Can you work these out from the model? Positions are in its coordinate system, mm. A direction names the side the tool comes from. Give positions to 0.01 mm unless a question says otherwise; leave off trailing zeros. Write each loop counter-clockwise with the first axis right and the second up, starting at its lowest first coordinate (ties: lowest second). Pieces come first, ordered by that corner, then holes. Notation, with made-up numbers: (62.25, -34) -> (119.25, -34) arc R19 ccw to (119.25, 2) -> close; hole circle Ø7 at (25.25, 2). An arc over 180 degrees is marked (long way). One line per item, written item: value.
from build123d import *

# Parameters (mm, degrees)
SKETCH1_W                                   = 100
SKETCH1_H                                   = 100
BOSS_EXTRUDE1_DEPTH                         = 6.5
SKETCH2_W                                   = 100
SKETCH2_H                                   = 100
BOSS_EXTRUDE2_DEPTH                         = 5
SKETCH3_W                                   = 100
SKETCH3_H                                   = 100
BOSS_EXTRUDE3_DEPTH                         = 5
CUT_EXTRUDE1_DEPTH                          = 101
SKETCH6_W                                   = 100
SKETCH6_H                                   = 100
SKETCH6_W_2                                 = 90
SKETCH6_H_2                                 = 90
CUT_EXTRUDE2_DEPTH                          = 5
SKETCH9_W                                   = 70
SKETCH9_H                                   = 70
BOSS_EXTRUDE4_DEPTH                         = 3.5
CBORE_FOR_M5_CHEESE_HEAD_SCREW1_D           = 3.332
CBORE_FOR_M5_CHEESE_HEAD_SCREW1_DEPTH       = 11
CBORE_FOR_M5_CHEESE_HEAD_SCREW1_CBORE_D     = 8
CBORE_FOR_M5_CHEESE_HEAD_SCREW1_CBORE_DEPTH = 5
CBORE_FOR_M5_CHEESE_HEAD_SCREW1_TIP         = 1.001033791
FILLET1_R                                   = 6.35
CHAMFER1_SIZE                               = 6.35
SKETCH14_W                                  = 25
SKETCH14_H                                  = 50
CUT_EXTRUDE3_DEPTH                          = 5


with BuildPart() as part:
    # Sketch1 → Boss-Extrude1 (new body)
    with BuildSketch(Plane(origin=(0, 0, 0), x_dir=(1, 0, 0), z_dir=(0, 1, 0))):
        Rectangle(SKETCH1_W, SKETCH1_H)
    extrude(amount=BOSS_EXTRUDE1_DEPTH)



with BuildPart() as body_2:
    # Sketch2 → Boss-Extrude2 (new body)
    with BuildSketch(Plane(origin=(0, -3.5, 0), x_dir=(-1, 0, 0), z_dir=(0, -1, 0))):
        Rectangle(SKETCH2_W, SKETCH2_H)
    extrude(amount=BOSS_EXTRUDE2_DEPTH)

    # Sketch3 → Boss-Extrude3 (add)
    with BuildSketch(Plane.XZ.offset(8.5)):
        Rectangle(SKETCH3_W, SKETCH3_H)
    extrude(amount=BOSS_EXTRUDE3_DEPTH)

    # Sketch4 → Cut-Extrude1 (cut, through all)
    with BuildSketch(Plane.XY.offset(50)):
        Polygon((-25, -13.5), (-25, -8.5), (-5, -8.5), (-7.886751346, -13.5), align=None)
    cut_extrude1 = extrude(amount=-CUT_EXTRUDE1_DEPTH, mode=Mode.SUBTRACT)

    # Mirror1: Cut-Extrude1 across plane
    add(cut_extrude1.mirror(Plane(origin=(0, 0, 0), x_dir=(0, 0, 1), z_dir=(1, 0, 0))), mode=Mode.SUBTRACT)

    # Sketch6 → Cut-Extrude2 (cut)
    with BuildSketch(Plane.XZ.offset(13.5)):
        Rectangle(SKETCH6_W, SKETCH6_H)
        Rectangle(SKETCH6_W_2, SKETCH6_H_2, mode=Mode.SUBTRACT)
    extrude(amount=-CUT_EXTRUDE2_DEPTH, mode=Mode.SUBTRACT)


with BuildPart() as part_1:
    add(part.part)

    add(body_2.part)  # Boss-Extrude4 merges body 2
    # Sketch9 → Boss-Extrude4 (add)
    with BuildSketch(Plane.XZ):
        Rectangle(SKETCH9_W, SKETCH9_H)
    extrude(amount=BOSS_EXTRUDE4_DEPTH)

    # CBORE for M5 Cheese Head Screw1
    with Locations(Plane(origin=(0, -13.5, 0), x_dir=(-1, 0, 0), z_dir=(0, -1, 0))):
        with Locations((-32, 32), (0, 32), (32, 32), (32, -32), (0, -32), (-32, -32)):
            CounterBoreHole(CBORE_FOR_M5_CHEESE_HEAD_SCREW1_D / 2, CBORE_FOR_M5_CHEESE_HEAD_SCREW1_CBORE_D / 2, CBORE_FOR_M5_CHEESE_HEAD_SCREW1_CBORE_DEPTH, depth=CBORE_FOR_M5_CHEESE_HEAD_SCREW1_DEPTH)
            with Locations((0, 0, -(CBORE_FOR_M5_CHEESE_HEAD_SCREW1_DEPTH + CBORE_FOR_M5_CHEESE_HEAD_SCREW1_TIP / 2))):  # 118° drill point
                Cone(0, CBORE_FOR_M5_CHEESE_HEAD_SCREW1_D / 2, CBORE_FOR_M5_CHEESE_HEAD_SCREW1_TIP, mode=Mode.SUBTRACT)

    # Fillet1
    fillet1_edges = [part_1.edges().sort_by_distance(p)[0] for p in [
        (50, -6, 50),
        (-50, -6, -50),
        (-50, -6, 50),
        (50, -6, -50),
        (-50, 3.25, -50),
        (50, 3.25, -50),
        (50, 3.25, 50),
        (-50, 3.25, 50),
    ]]
    fillet(fillet1_edges, radius=FILLET1_R)

    # Chamfer1
    chamfer1_edges = [part_1.edges().sort_by_distance(p)[0] for p in [
        (45, -11, -45),
        (45, -11, 45),
        (-45, -11, 45),
        (-45, -11, -45),
    ]]
    chamfer(chamfer1_edges, length=CHAMFER1_SIZE)

    # Sketch14 → Cut-Extrude3 (cut)
    with BuildSketch(Plane.XZ.offset(13.5)):
        with Locations((-37.5, 0)):
            Rectangle(SKETCH14_W, SKETCH14_H)
    cut_extrude3 = extrude(amount=-CUT_EXTRUDE3_DEPTH, mode=Mode.SUBTRACT)

    # Mirror2: Cut-Extrude3 across plane
    add(cut_extrude3.mirror(Plane(origin=(0, 0, 0), x_dir=(0, 0, 1), z_dir=(1, 0, 0))), mode=Mode.SUBTRACT)


solid = part_1.part
1) For faces 4 (the face through (-25, -11, 35)), 5 (the face through (45, -11, 32)), 6 (the face through (32.521, -11.035, -35.966)), 7 (the face through (-35, -11, 25)), which set-ups out of +Z, -Z, +X, -X, +Y, -Y let a thin tool reach every point of the face, with its end or its side?
Answer list:
face 4: +Z, -Z, -Y
face 5: +Z, -Z, +X, -Y
face 6: -Y
face 7: -X, -Y
2) Will these pins go through, and if not, where does the flat tip stop? pin 1 (4 mm diameter, centred on x = -31, y = -11, fed in from +Z); pin 2 (5 mm diameter, centred on x = 32, z = 32, fed in from -Y); pin 3 (6.5 mm diameter, centred on x = 31, z = -33, fed in from -Y); pin 4 (1 mm diameter, centred on y = -2.5, z = -11, fed in from +X).
Answer list:
pin 1: stops at z = 45
pin 2: stops at y = -8.5
pin 3: stops at y = -13.5
pin 4: stops at x = 35
3) We'd pull the mould along X, two halves only. Please class faces 1 (the face through (50, -6, -1)), 2 (the face through (35, -13.5, -35)), 3 (the face through (25, -11, 35)): released by +X, released by -X, zero draft, split by the parting line, or undercut.
Answer list:
face 1: released by +X
face 2: zero draft
face 3: undercut
4) If we section it at A-A (z = 22.5): Write out the boundary of the cut face in (x, y).
Answer list:
outline: (-50, -8.5) -> (-5, -8.5) -> (-7.89, -13.5) -> (7.89, -13.5) -> (5, -8.5) -> (50, -8.5) -> (50, -3.5) -> (35, -3.5) -> (35, 0) -> (50, 0) -> (50, 6.5) -> (-50, 6.5) -> (-50, 0) -> (-35, 0) -> (-35, -3.5) -> (-50, -3.5) -> close
5) If we section it at B-B (x = -22): Write out the boundary of the cut face in (y, z).
Answer list:
outline: (-8.5, -50) -> (-3.5, -50) -> (-3.5, -35) -> (0, -35) -> (0, -50) -> (6.5, -50) -> (6.5, 50) -> (0, 50) -> (0, 35) -> (-3.5, 35) -> (-3.5, 50) -> (-8.5, 50) -> close
6) I need wall thicknesses on L1, parallel to X at y = -4.35, z = -32; L2, parallel to Z at x = 0, y = -12.3; L3, parallel to Z at x = 32, y = -5.55. Which ranges of each line are inside material? Lowest first, please.
Answer list:
L1: x = -50 to -33.67, -30.33 to -1.67, 1.67 to 30.33, 33.67 to 50
L2: z = -45 to -36, -28 to 28, 36 to 45
L3: z = -50 to -33.67, -30.33 to 30.33, 33.67 to 50
